```python
from build123d import *

# Parameters (mm, degrees)
SKETCH1_R                 = 1.984375
BOSS_EXTRUDE1_DEPTH       = 1.47955
F_4_CLEARANCE_HOLE1_D     = 2.9464
F_4_CLEARANCE_HOLE1_DEPTH = 3.302
F_4_CLEARANCE_HOLE1_TIP   = 0.885187864


with BuildPart() as part:
    # Sketch1 → Boss-Extrude1 (new body, symmetric)
    with BuildSketch(Plane.XY):
        with BuildLine():
            Line((-15.6591, -1.5875), (-15.6591, -7.9375))
            Line((-15.6591, -7.9375), (-12.7, -7.9375))
            Line((-12.7, -7.9375), (-12.7, -11.1125))
            Line((-12.7, -11.1125), (12.7, -11.1125))
            Line((12.7, -11.1125), (12.7, -7.9375))
            Line((12.7, -7.9375), (15.6591, -7.9375))
            Line((15.6591, -7.9375), (15.6591, -1.5875))
            Line((15.6591, -1.5875), (12.7, -1.5875))
            Line((12.7, -1.5875), (12.7, 1.5875))
            Line((12.7, 1.5875), (4.909072636, 1.5875))
            ThreePointArc((4.909072636, 1.5875), (0, 5.159375), (-4.909072636, 1.5875))
            Line((-4.909072636, 1.5875), (-12.7, 1.5875))
            Line((-12.7, 1.5875), (-12.7, -1.5875))
            Line((-12.7, -1.5875), (-15.6591, -1.5875))
        make_face()
        Circle(SKETCH1_R, mode=Mode.SUBTRACT)
    extrude(amount=BOSS_EXTRUDE1_DEPTH, both=True)

    # #4 Clearance Hole1
    with Locations(Plane(origin=(0.047806488, 1.573653324, 1.47955), x_dir=(1, 0, 0), z_dir=(0, 0, 1))):
        with Locations((-9.064806488, -6.336153324), (8.969193512, -6.336153324)):
            Hole(F_4_CLEARANCE_HOLE1_D / 2, depth=F_4_CLEARANCE_HOLE1_DEPTH)
            with Locations((0, 0, -(F_4_CLEARANCE_HOLE1_DEPTH + F_4_CLEARANCE_HOLE1_TIP / 2))):  # 118° drill point
                Cone(0, F_4_CLEARANCE_HOLE1_D / 2, F_4_CLEARANCE_HOLE1_TIP, mode=Mode.SUBTRACT)


solid = part.part
```
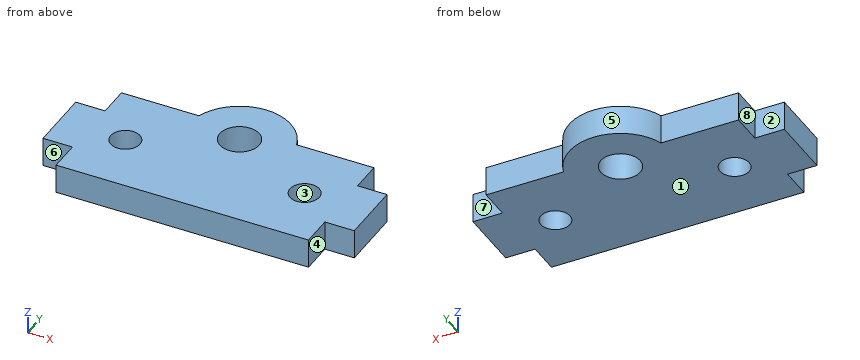
The listing builds one solid part. Answer for the finished solid, in the listing's coordinates (mm). Face numbers are marked on the shaded views. A direction names the side the tool comes from. Coordinates: 2 decimals unless noted, no trailing zeros. Write each loop counter-clockwise with the first axis right and the second up, starting at its lowest first coordinate (ties: lowest second). Pieces come first, ordered by that corner, then holes.
Q1. Section D-D, the plane y = -9.5 is taken. Write down the section's boundary in (x, z).
Returned:
outline: (-12.7, -1.48) - (12.7, -1.48) - (12.7, 1.48) - (-12.7, 1.48) - close
Q2. Given P1, Ø3.5, axis at x = 9.02, y = -4.76, coming from the -Z side; P2, Ø1.5, axis at y = 0.5, z = 0, coming from the +X side; P3, Ø1, axis at x = 10, y = 2.5, coming from the -Z side; P4, Ø1, axis at x = -7.5, z = -1, coming from the +Y side, each flat-ended and moving along its own axis, determine where each tip first touches the part or whether it passes through.
Returned:
P1: stops at z = -1.48
P2: stops at x = 12.7
P3: passes through
P4: stops at y = 1.59
Q3. The mould has two halves that part along Y. Classify the marked faces 1, 2 and 3: released by +Y, released by -Y, zero draft, split by the parting line, or undercut.
Returned:
face 1: zero draft
face 2: released by +Y
face 3: undercut
Q4. Section C-C, the plane z = 0.05 is taken. Write down the section's boundary in (x, y), then the cut area to 3 significant figures.
Returned:
outline: (-15.66, -7.94) - (-12.7, -7.94) - (-12.7, -11.11) - (12.7, -11.11) - (12.7, -7.94) - (15.66, -7.94) - (15.66, -1.59) - (12.7, -1.59) - (12.7, 1.59) - (4.91, 1.59) arc R5.16 ccw to (-4.91, 1.59) - (-12.7, 1.59) - (-12.7, -1.59) - (-15.66, -1.59) - close; hole circle Ø2.95 at (-9.02, -4.76); hole circle Ø3.97 at (0, 0); hole circle Ø2.95 at (9.02, -4.76)
area: 360 mm2
Q5. Section B-B, the plane x = 0 is taken. Write down the section's boundary in (y, z).
Returned:
outline: (-11.11, -1.48) - (-1.98, -1.48) - (-1.98, 1.48) - (-11.11, 1.48) - close; (1.98, -1.48) - (5.16, -1.48) - (5.16, 1.48) - (1.98, 1.48) - close
Q6. Section A-A, the plane y = 0 is taken. Write down the section's boundary in (x, z), then the cut area to 3 significant figures.
Returned:
outline: (-12.7, -1.48) - (-1.98, -1.48) - (-1.98, 1.48) - (-12.7, 1.48) - close; (1.98, -1.48) - (12.7, -1.48) - (12.7, 1.48) - (1.98, 1.48) - close
area: 63.4 mm2
Q7. Which of the six approach directions +Z, -Z, +X, -X, +Y, -Y give full straight-line access (tool end or side, diameter ignored) to the marked faces 4, 5, 6, 7 and 8?
Returned:
face 4: +Z, -Z, +X, -Y
face 5: +Z, -Z, +Y
face 6: +Z, -Z, -X, -Y
face 7: +Z, -Z, +X, +Y
face 8: +Z, -Z, -X, +Y
Q8. Find the intervals of material crossed by line 1 along X through (y, z) = (-3.5, -0.35); line 2 along X through (y, z) = (-4, -0.25); line 3 along Y through (x, z) = (9, 1.1), in increasing order.
Returned:
line 1: x = -15.66 to -9.78, -8.26 to 8.26, 9.78 to 15.66
line 2: x = -15.66 to -10.28, -7.76 to 7.76, 10.28 to 15.66
line 3: y = -11.11 to -6.24, -3.29 to 1.59
